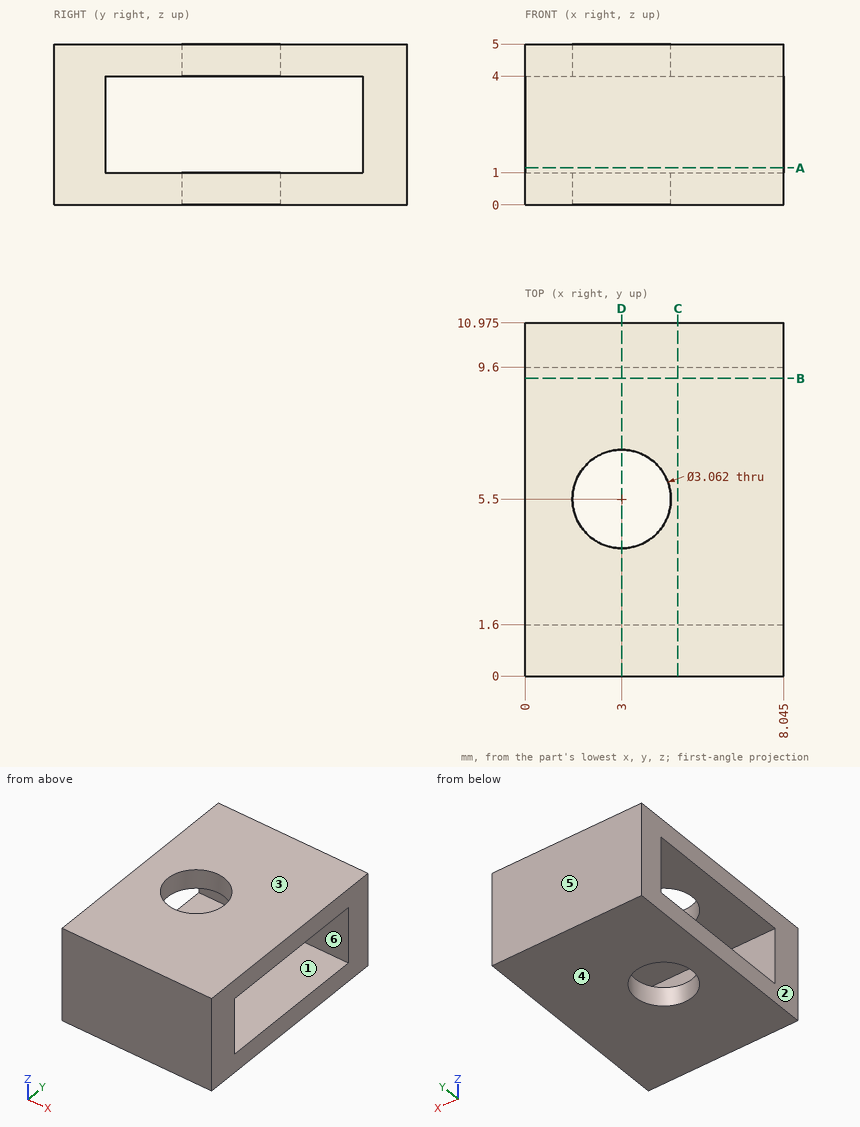
Answer from the drawing. Dimensions are ordinates in mm from the lowest x, y and z of the part. A direction names the side the tool comes from. Round coordinates to 2 decimals unless told otherwise and drop trailing zeros. Loops run counter-clockwise (first coordinate to the right, second up) from the corner with the lowest first, then second, coordinate; pieces in that order, holes last. Notation, with made-up numbers: (-25.75, 70.5) - (-13.75, 70.5) arc R24 cw to (-13.75, 80.5) - close; hole circle Ø10 at (-27, 66). An arc over 180 degrees is marked (long way). One line per item, written item: value.
Q1. The mould has two halves that part along Z. Classify the marked faces 1, 2, 3 and 4: +Z half, -Z half, draft (parallel to the pull), parting line (faces both ways), or undercut.
Check values:
face 1: undercut
face 2: draft
face 3: +Z half
face 4: -Z half
Q2. Each of these flat-tipped pins is pushed along its axis until it touches: pin 1 Ø1.5 at (x, y) = (3.5, 8.5) entering from -Z; pin 2 Ø1.8 at (x, y) = (3, 5.5) entering from +Z. Where does it stop, or does it pass through?
Check values:
pin 1: z = 0
pin 2: through
Q3. Straight lines are drawn through the part: probe 1 along Y at (x, z) = (3.5, 2.5) (1 decimal); probe 2 along Z at (x, y) = (0.5, 6.5); probe 3 along Y at (x, z) = (3.25, 0.8) (1 decimal). For each, find the intervals that lie inside material, in ascending order.
Check values:
probe 1: 0 to 1.6, 9.6 to 11
probe 2: 0 to 1, 4 to 5
probe 3: 0 to 4, 7 to 11
Q4. Find section C-C on x = 4.75. Give the vertices of the cut face in (y, z) (1 decimal).
Check values:
outline: (0, 0) - (11, 0) - (11, 5) - (0, 5) - close; hole (1.6, 1) - (9.6, 1) - (9.6, 4) - (1.6, 4) - close
Q5. For the marked faces 5 and 6, determine the directions among +Z, -Z, +X, -X, +Y, -Y from which every point of the face is accessible in a straight line to the end or side of a thin tool.
Check values:
face 5: +Z, -Z, +X, -X, +Y
face 6: +X, -X
Q6. Find section A-A on z = 1.15. Give the vertices of the cut face in (x, y) (1 decimal).
Check values:
outline: (0, 0) - (8, 0) - (8, 1.6) - (0, 1.6) - close; (0, 9.6) - (8, 9.6) - (8, 11) - (0, 11) - close
Q7. Find section B-B on y = 9.25. Give the vertices of the cut face in (x, z) (1 decimal), and give its area (3 significant figures).
Check values:
outline: (0, 0) - (8, 0) - (8, 1) - (0, 1) - close; (0, 4) - (8, 4) - (8, 5) - (0, 5) - close
area: 16.1 mm2
Q8. Find section D-D on x = 3. Give the vertices of the cut face in (y, z) (1 decimal).
Check values:
outline: (0, 0) - (4, 0) - (4, 1) - (1.6, 1) - (1.6, 4) - (4, 4) - (4, 5) - (0, 5) - close; (7, 0) - (11, 0) - (11, 5) - (7, 5) - (7, 4) - (9.6, 4) - (9.6, 1) - (7, 1) - close
